The listing builds one solid part. Answer for the finished solid, in the listing's coordinates (mm). Face numbers are marked on the shaded views. A direction names the side the tool comes from. Coordinates: 2 decimals unless noted, no trailing zeros. Write each loop counter-clockwise with the first axis right and the second up, starting at its lowest first coordinate (ties: lowest second). Pieces come first, ordered by that corner, then holes.
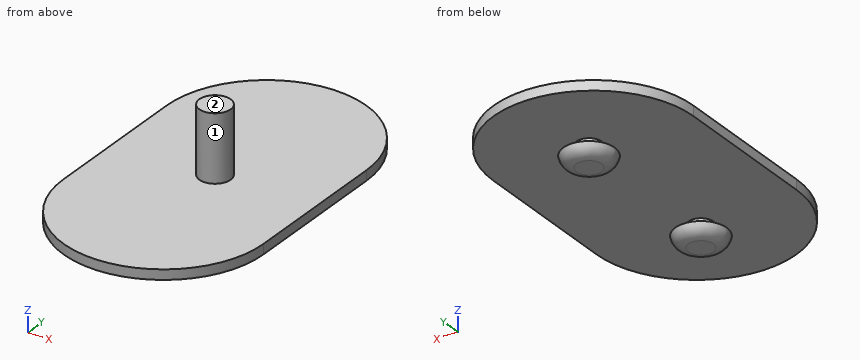
from build123d import *

# Parameters (mm, degrees)
DODANIE_WYCI_GNI_CIE2_DEPTH = 1.5
SZKIC37_R                   = 1.85
DODANIE_WYCI_GNI_CIE3_DEPTH = 1.5
SZKIC38_R                   = 3.85
DODANIE_WYCI_GNI_CIE4_DEPTH = 1.7
ZAOKR_GLENIE1_R             = 2
SZKIC39_R                   = 2.35
DODANIE_WYCI_GNI_CIE5_DEPTH = 10


with BuildPart() as part:
    # Szkic35 → Dodanie-wyciągnięcie2 (new body)
    with BuildSketch(Plane.XY):
        with BuildLine():
            Line((-15, -11.5), (-15, 11.5))
            ThreePointArc((-15, 11.5), (0, 26.5), (15, 11.5))
            Line((15, 11.5), (15, -11.5))
            ThreePointArc((15, -11.5), (0, -26.5), (-15, -11.5))
        make_face()
    extrude(amount=DODANIE_WYCI_GNI_CIE2_DEPTH)

    # Szkic37 → Dodanie-wyciągnięcie3 (add)
    with BuildSketch(Plane(origin=(0, 0, 0), x_dir=(-1, 0, 0), z_dir=(0, 0, -1))):
        with Locations((0, 12.5)):
            Circle(SZKIC37_R)
        with Locations((0, -12.5)):
            Circle(SZKIC37_R)
    extrude(amount=DODANIE_WYCI_GNI_CIE3_DEPTH)

    # Szkic38 → Dodanie-wyciągnięcie4 (add)
    with BuildSketch(Plane(origin=(0, 0, -1.5), x_dir=(-1, 0, 0), z_dir=(0, 0, -1))):
        with Locations((0, 12.5)):
            Circle(SZKIC38_R)
        with Locations((0, -12.5)):
            Circle(SZKIC38_R)
    extrude(amount=DODANIE_WYCI_GNI_CIE4_DEPTH)

    # Zaokrąglenie1
    # the kernel refuses this fillet: 2 mm, written as the material it takes off along each edge
    with BuildSketch(Plane(origin=(0, 12.5, -3.2), x_dir=(-1, 0, 0), z_dir=(0, -1, 0))) as zaokr_glenie1_piece_1:
        with BuildLine():
            CenterArc((1.872628007, -2), ZAOKR_GLENIE1_R, 8.626926559, 81.373073441)
            Line((1.872628007, 0), (1.872628007, 0.04))
            Line((1.872628007, 0.04), (3.85, 0.04))
            Line((3.85, 0.04), (3.89, 0))
            ThreePointArc((3.89, 0), (3.89, -0.85), (3.88954744, -1.694))
            Line((3.88954744, -1.694), (3.85, -1.7))
        make_face()
    revolve(axis=Axis((0, 12.5, -3.2), (0, 0, -1)), mode=Mode.SUBTRACT)
    with BuildSketch(Plane(origin=(0, -12.5, -3.2), x_dir=(-1, 0, 0), z_dir=(0, -1, 0))) as zaokr_glenie1_piece_2:
        with BuildLine():
            CenterArc((1.872628007, -2), ZAOKR_GLENIE1_R, 8.626926559, 81.373073441)
            Line((1.872628007, 0), (1.872628007, 0.04))
            Line((1.872628007, 0.04), (3.85, 0.04))
            Line((3.85, 0.04), (3.89, 0))
            ThreePointArc((3.89, 0), (3.89, -0.85), (3.88954744, -1.694))
            Line((3.88954744, -1.694), (3.85, -1.7))
        make_face()
    revolve(axis=Axis((0, -12.5, -3.2), (0, 0, -1)), mode=Mode.SUBTRACT)

    # Szkic39 → Dodanie-wyciągnięcie5 (add)
    with BuildSketch(Plane.XY.offset(1.5)):
        with Locations(Location((0, 0, 0), (0, 0, 180))):
            Circle(SZKIC39_R)
    extrude(amount=DODANIE_WYCI_GNI_CIE5_DEPTH)


solid = part.part
Q1. The part is cut by section C-C, the plane y = 6. Write down the section's boundary in (x, z), then the cut area to 3 significant figures.
Answers below:
outline: (-15, 0) - (15, 0) - (15, 1.5) - (-15, 1.5) - close
area: 45.0 mm2
Q2. Given pin 1 (8.5 mm diameter, centred on x = 1, y = 13.5, fed in from +Z); pin 2 (1 mm diameter, centred on y = 19.5, z = 1, fed in from +X); pin 3 (4 mm diameter, centred on x = 8, y = 20, fed in from -Z), each flat-ended and moving along its own axis, determine where each tip first touches the part or whether it passes through.
Answers below:
pin 1: stops at z = 1.5
pin 2: stops at x = 12.99
pin 3: stops at z = 0
Q3. Which of the six approach directions +Z, -Z, +X, -X, +Y, -Y give full straight-line access (tool end or side, diameter ignored) to the marked faces 1 and 2?
Answers below:
face 1: +Z
face 2: +Z, +X, -X, +Y, -Y
Q4. Find the intervals of material crossed by probe 1 along Z at (x, y) = (-1, 17); probe 2 along Z at (x, y) = (-1, -2); probe 3 along Y at (x, z) = (1.5, 0.25), in increasing order.
Answers below:
probe 1: z = 0 to 1.5
probe 2: z = 0 to 11.5
probe 3: y = -26.42 to 26.42
Q5. The part is cut by section A-A, the plane z = 8.5. Write down the section's boundary in (x, y).
Answers below:
outline: circle Ø4.7 at (0, 0)
Q6. The part is cut by section B-B, the plane x = -3. State how many separate pieces and enclosed holes the cut face has, then the cut area to 3 significant figures.
Answers below:
separate pieces: 3
enclosed holes: 0
area: 88.6 mm2
Q7. The part is cut by section D-D, the plane x = -7. Write down the section's boundary in (y, z).
Answers below:
outline: (-24.77, 0) - (24.77, 0) - (24.77, 1.5) - (-24.77, 1.5) - close
